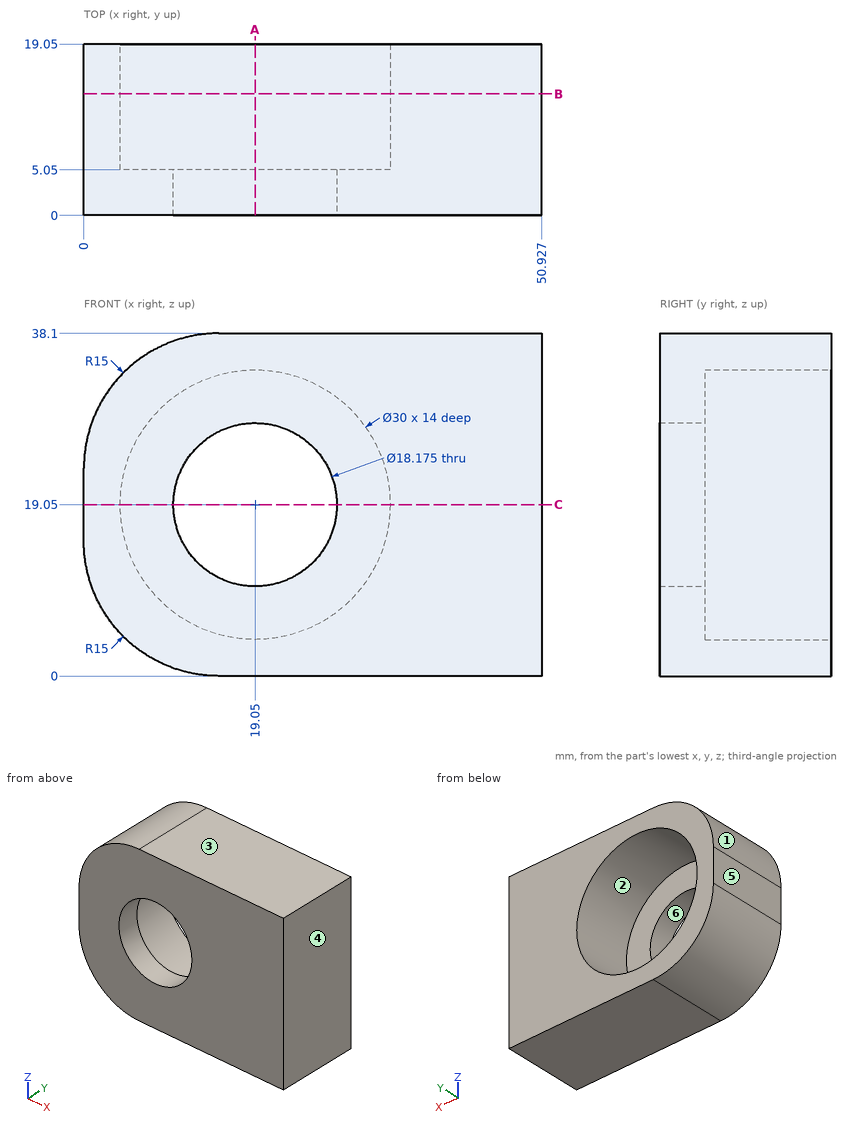
Answer from the drawing. Dimensions are ordinates in mm from the lowest x, y and z of the part. A direction names the side the tool comes from. Coordinates: 2 decimals unless noted, no trailing zeros. Write each loop counter-clockwise with the first axis right and the second up, starting at its lowest first coordinate (ties: lowest second). Pieces come first, ordered by that corner, then holes. Notation, with made-up numbers: M -19.5,-11 L 6.5,-11 A30 cw 6.5,15 Z; hole C -11,68.5 d5. An arc over 180 degrees is marked long. Write item = value, one per line.
1. For the marked faces 1 and 2, determine the directions among +Z, -Z, +X, -X, +Y, -Y from which every point of the face is accessible in a straight line to the end or side of a thin tool.
Solution:
face_1 = +Z, -X, +Y, -Y
face_2 = +Y
2. The part is cut by section A-A (x = 19.05). Determine the outline of the cut face in (y, z).
Solution:
outline = M 0,0 L 19.05,0 L 19.05,4.05 L 5.05,4.05 L 5.05,9.96 L 0,9.96 Z; M 0,28.14 L 5.05,28.14 L 5.05,34.05 L 19.05,34.05 L 19.05,38.1 L 0,38.1 Z
3. Straight lines are drawn through the part: line 1 (X direction, y = 13.75, z = 19.05); line 2 (Z direction, x = 19.05, y = 11); line 3 (Z direction, x = 19.05, y = 1.4). For each, find the intervals that lie inside material, in ascending order. Write a range as from..to.
Solution:
line_1 = 0..4.05, 34.05..50.93
line_2 = 0..4.05, 34.05..38.1
line_3 = 0..9.96, 28.14..38.1
4. The part is cut by section C-C (z = 19.05). Determine the outline of the cut face in (x, y), then the cut area to 3 significant figures.
Solution:
outline = M 0,0 L 9.96,0 L 9.96,5.05 L 4.05,5.05 L 4.05,19.05 L 0,19.05 Z; M 28.14,0 L 50.93,0 L 50.93,19.05 L 34.05,19.05 L 34.05,5.05 L 28.14,5.05 Z
area = 458 mm2
5. The part is cut by section B-B (y = 13.5). Determine the outline of the cut face in (x, z).
Solution:
outline = M 0,15 A15 ccw 15,0 L 50.93,0 L 50.93,38.1 L 15,38.1 A15 ccw 0,23.1 Z; hole C 19.05,19.05 d30
6. Determine the mould class of the marked faces 3, 4, 5 and 6 for opening direction X: released by +X, released by -X, zero draft, split by the parting line, or undercut.
Solution:
face_3 = zero draft
face_4 = released by +X
face_5 = released by -X
face_6 = undercut
7. Flat-ended cylindrical pins translate along their axes: pin 1 (6 mm diameter, centred on y = 11.5, z = 31, fed in from -X); pin 2 (1.5 mm diameter, centred on x = 16, y = 15.5, fed in from -Z). Find the tip coordinate at first contact, or state that the pin passes through.
Solution:
pin_1 = 0.82
pin_2 = 0
